The figure shows three views and two pictorial views of one solid part (mm, origin at its lowest corner). Answer the questions. Give positions to 0.01 mm unless a question says otherwise; leave off trailing zeros. Write each loop counter-clockwise with the first axis right and the second up, starting at its lowest first coordinate (ties: lowest second). Pieces come first, ordered by that corner, then holes. Notation, with made-up numbers: (47, 2.25) -> (74, 2.25) arc R17 cw to (74, 31.25) -> close; hole circle Ø6 at (78.25, 41.25). An arc over 180 degrees is marked (long way). Use a Markdown table: item, result.
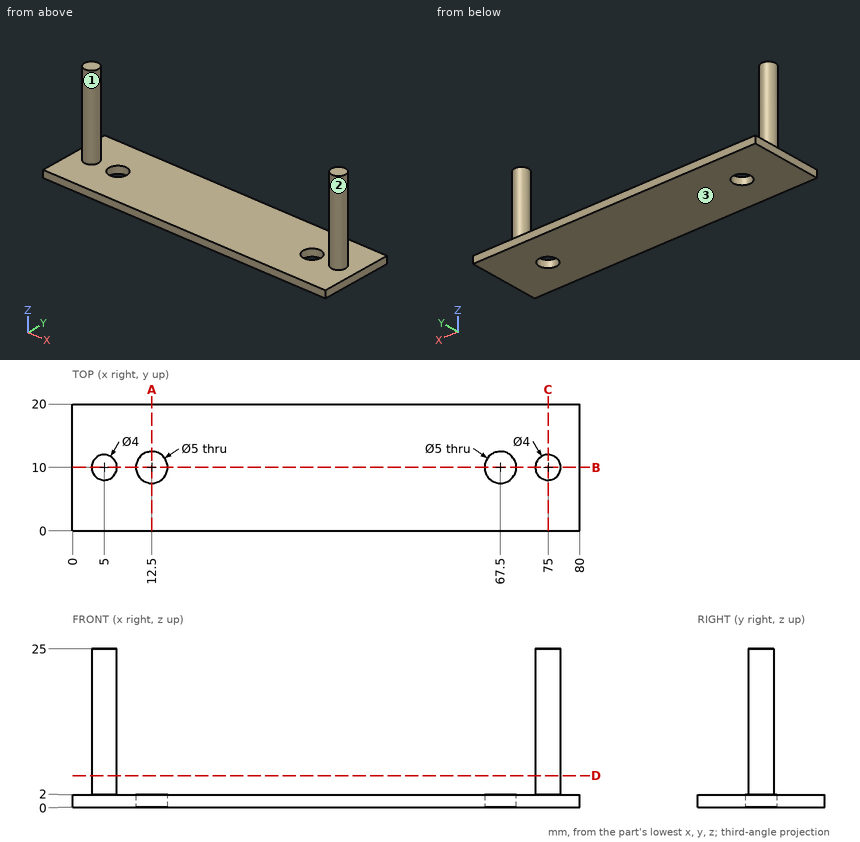
Item 1: For a pull along X with two mould halves and no side action, classify the marked faces 1, 2 and 3 as +X half, -X half, draft (parallel to the pull), parting line (faces both ways), or undercut.
Return value:
| item | result |
|---|---|
| face 1 | undercut |
| face 2 | undercut |
| face 3 | draft |
Item 2: A cutting plane is placed at A-A (x = 12.5). Give the vertices of the cut face in (y, z).
Return value:
| item | result |
|---|---|
| outline | (0, 0) -> (7.5, 0) -> (7.5, 2) -> (0, 2) -> close; (12.5, 0) -> (20, 0) -> (20, 2) -> (12.5, 2) -> close |
Item 3: A cutting plane is placed at D-D (z = 5). Give the vertices of the cut face in (x, y).
Return value:
| item | result |
|---|---|
| outline | circle Ø4 at (5, 10); circle Ø4 at (75, 10) |
Item 4: A cutting plane is placed at B-B (y = 10). Give the vertices of the cut face in (x, z).
Return value:
| item | result |
|---|---|
| outline | (0, 0) -> (10, 0) -> (10, 2) -> (7, 2) -> (7, 25) -> (3, 25) -> (3, 2) -> (0, 2) -> close; (15, 0) -> (65, 0) -> (65, 2) -> (15, 2) -> close; (70, 0) -> (80, 0) -> (80, 2) -> (77, 2) -> (77, 25) -> (73, 25) -> (73, 2) -> (70, 2) -> close |
Item 5: Each of these flat-tipped pins is pushed along its axis until it touches: P1, Ø3, axis at y = 16.5, z = 4, coming from the -X side (3 decimals); P2, Ø6, axis at x = 67.5, y = 10, coming from the +Z side; P3, Ø6.5, axis at x = 12.5, y = 10, coming from the -Z side; P4, Ø5, axis at y = 14, z = 16.5, coming from the +X side. Where does it stop, or does it pass through?
Return value:
| item | result |
|---|---|
| P1 | through |
| P2 | z = 2 |
| P3 | z = 0 |
| P4 | x = 76.32 |
Item 6: A cutting plane is placed at C-C (x = 75). Give the vertices of the cut face in (y, z).
Return value:
| item | result |
|---|---|
| outline | (0, 0) -> (20, 0) -> (20, 2) -> (12, 2) -> (12, 25) -> (8, 25) -> (8, 2) -> (0, 2) -> close |
Item 7: Straight lines are drawn through the part: line 1 along Y through (x, z) = (12.5, 1.3); line 2 along Z through (x, y) = (67, 13); line 3 along X through (y, z) = (8.5, 1.5). For each, find the intervals that lie inside material, in ascending order. Write a range as [from, to].
Return value:
| item | result |
|---|---|
| line 1 | [0, 7.5], [12.5, 20] |
| line 2 | [0, 2] |
| line 3 | [0, 10.5], [14.5, 65.5], [69.5, 80] |
